Design review of the part built by this model. Coordinates are the model's own, in mm. Face numbers are marked on the shaded views. A direction names the side the tool comes from. Round coordinates to 2 decimals unless told otherwise and drop trailing zeros. Loops run counter-clockwise (first coordinate to the right, second up) from the corner with the lowest first, then second, coordinate; pieces in that order, holes last. Notation, with made-up numbers: (-28.5, 82.25) - (-6.5, 82.25) arc R10 cw to (-6.5, 100.25) - close; hole circle Ø6 at (-25.75, 36.5). An arc over 180 degrees is marked (long way). Return JSON: item names as keys, results as strings. Group by question number.
(1) The part is to be moulded in two halves that separate along X. For the marked faces 3, 4 and 5, say which applies: pulls with the +X half, pulls with the -X half, needs draft (parallel to the pull), parting line crosses it, or undercut.
(2) We need section D-D, the plane z = -13.5. Write out the cut boundary in (x, y), and give its area (3 significant figures).
(3) We need section B-B, the plane y = 20.25. Write out the cut boundary in (x, z).
(4) Wall thickness on L1, parallel to X at y = 25.7, z = 13.5; L2, parallel to X at y = 5, z = -13.5; L3, parallel to X at y = 9, z = 0: over which ranges is each line inside the solid? List them lowest first. Write a range as [from, to].
(5) For the marked faces 1 and 2, list the 3-axis set-ups (+Z, -Z, +X, -X, +Y, -Y) from which the entire face can be reached by the end or side of a thin tool; tool diameter is ignored.
(6) We need section A-A, the plane z = 0. Write out the cut boundary in (x, y).
(7) We need section C-C, the plane x = 0. Give the number of separate pieces and of enclosed holes in the cut face, and give its area (3 significant figures).
(8) Clearance check with flat-ended pins moving along their axes: pin 1 (1.5 mm diameter, centred on y = 20, z = -22.5, fed in from +X); pin 2 (11 mm diameter, centred on x = -2, z = -29, fed in from +Y); pin 3 (10 mm diameter, centred on x = 8.5, z = -0.5, fed in from +Y); pin 4 (10 mm diameter, centred on y = 26, z = -17, fed in from -X). State where each tip first meets the part, or that it passes through.
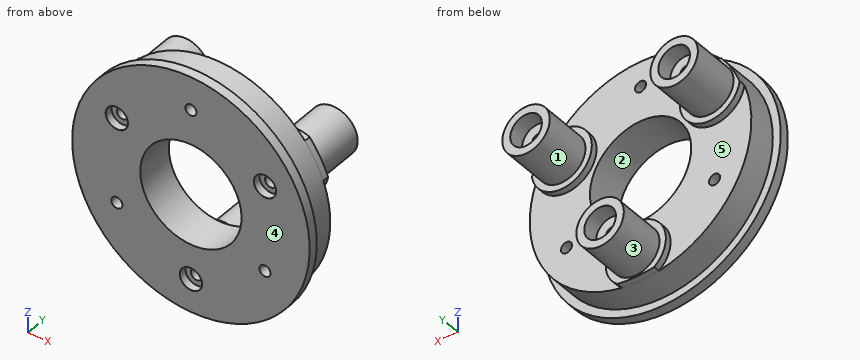
from build123d import *

# Parameters (mm, degrees)
SKETCH1_R                                     = 37.5
BOSS_EXTRUDE1_DEPTH                           = 3
SKETCH1_3_R                                   = 35
BOSS_EXTRUDE2_DEPTH                           = 12
SKETCH13_R                                    = 16
CUT_EXTRUDE6_DEPTH                            = 55.373706881
BOSS_EXTRUDE9_DEPTH                           = 2
SKETCH25_R                                    = 7.5
BOSS_EXTRUDE10_DEPTH                          = 15
SKETCH26_R                                    = 5
CUT_EXTRUDE9_DEPTH                            = 5
CBORE_FOR_M3_PAN_HEAD_MACHINE_SCREW1_AT_COUNT = 2
CBORE_FOR_M3_PAN_HEAD_MACHINE_SCREW1_AT_PITCH = 46.765371804
CBORE_FOR_M3_PAN_HEAD_MACHINE_SCREW1_2_COUNT  = 2
CBORE_FOR_M3_PAN_HEAD_MACHINE_SCREW1_2_PITCH  = 46.765371804
SKETCH29_R                                    = 1.75
CUT_EXTRUDE10_DEPTH                           = 56.691112397


with BuildPart() as part:
    # Sketch1 → Boss-Extrude1 (new body)
    with BuildSketch(Plane(origin=(0, 0, 0), x_dir=(1, 0, 0), z_dir=(0, 1, 0))):
        with Locations(Location((0, 0, 0), (0, 0, 270))):
            Circle(SKETCH1_R)
    extrude(amount=BOSS_EXTRUDE1_DEPTH)

    # Sketch1_3 → Boss-Extrude2 (add)
    with BuildSketch(Plane(origin=(0, 0, 0), x_dir=(1, 0, 0), z_dir=(0, 1, 0))):
        with Locations(Location((0, 0, 0), (0, 0, 270))):
            Circle(SKETCH1_3_R)
    extrude(amount=BOSS_EXTRUDE2_DEPTH)

    # Sketch13 → Cut-Extrude6 (cut, through all)
    with BuildSketch(Plane(origin=(0, 12, 0), x_dir=(1, 0, 0), z_dir=(0, 1, 0))):
        with Locations(Location((0, 0, 0), (0, 0, 270))):
            Circle(SKETCH13_R)
    extrude(amount=-CUT_EXTRUDE6_DEPTH, mode=Mode.SUBTRACT)

    # Sketch24 → Boss-Extrude9 (add)
    with BuildSketch(Plane(origin=(0, 12, 0), x_dir=(1, 0, 0), z_dir=(0, 1, 0))):
        with BuildLine():
            ThreePointArc((5.813043417, 34.513888889), (0, 35), (-5.813043417, 34.513888889))
            ThreePointArc((-5.813043417, 34.513888889), (0, 17.5), (5.813043417, 34.513888889))
        make_face()
        with BuildLine():
            ThreePointArc((-26.983382853, -22.291187717), (-15.155444566, -8.75), (-32.79642627, -12.222701172))
            ThreePointArc((-32.79642627, -12.222701172), (-30.310889132, -17.5), (-26.983382853, -22.291187717))
        make_face()
        with BuildLine():
            ThreePointArc((26.983382853, -22.291187717), (30.310889132, -17.5), (32.79642627, -12.222701172))
            ThreePointArc((32.79642627, -12.222701172), (15.155444566, -8.75), (26.983382853, -22.291187717))
        make_face()
    extrude(amount=BOSS_EXTRUDE9_DEPTH)

    # Sketch25 → Boss-Extrude10 (add)
    with BuildSketch(Plane(origin=(0, 14, 0), x_dir=(1, 0, 0), z_dir=(0, 1, 0))):
        with Locations(Location((0, 27, 0), (0, 0, 270))):
            Circle(SKETCH25_R)
        with Locations(Location((23.382685902, -13.5, 0), (0, 0, 270))):
            Circle(SKETCH25_R)
        with Locations(Location((-23.382685902, -13.5, 0), (0, 0, 270))):
            Circle(SKETCH25_R)
    extrude(amount=BOSS_EXTRUDE10_DEPTH)

    # Sketch26 → Cut-Extrude9 (cut)
    with BuildSketch(Plane(origin=(0, 29, 0), x_dir=(1, 0, 0), z_dir=(0, 1, 0))):
        with Locations(Location((0, 27, 0), (0, 0, 270))):
            Circle(SKETCH26_R)
        with Locations(Location((23.382685902, -13.5, 0), (0, 0, 270))):
            Circle(SKETCH26_R)
        with Locations(Location((-23.382685902, -13.5, 0), (0, 0, 270))):
            Circle(SKETCH26_R)
    extrude(amount=-CUT_EXTRUDE9_DEPTH, mode=Mode.SUBTRACT)

    # Sketch28 → CBORE for M3 Pan Head Machine Screw1 (revolve, cut)
    with BuildSketch(Plane(origin=(0, 0, -27), x_dir=(0, 0, -1), z_dir=(1, 0, 0))):
        Polygon((0, 0), (0, 29), (1.8, 29), (1.8, 2.4), (3.5, 2.4), (3.5, 0.025), (3.525, 0), align=None)
    cbore_for_m3_pan_head_machine_screw1 = revolve(axis=Axis((0, -6.35, -27), (0, 1, 0)), mode=Mode.SUBTRACT)

    # CBORE for M3 Pan Head Machine Screw1 at: CBORE for M3 Pan Head Machine Screw1 ×2
    with Locations(*[Vector(-0.5000000000000369, 0, 0.8660254037844174) * (i * CBORE_FOR_M3_PAN_HEAD_MACHINE_SCREW1_AT_PITCH) for i in range(1, CBORE_FOR_M3_PAN_HEAD_MACHINE_SCREW1_AT_COUNT)]):
        add(cbore_for_m3_pan_head_machine_screw1, mode=Mode.SUBTRACT)

    # CBORE for M3 Pan Head Machine Screw1 2: CBORE for M3 Pan Head Machine Screw1 ×2
    with Locations(*[Vector(0.49999999999996353, 0, 0.8660254037844598) * (i * CBORE_FOR_M3_PAN_HEAD_MACHINE_SCREW1_2_PITCH) for i in range(1, CBORE_FOR_M3_PAN_HEAD_MACHINE_SCREW1_2_COUNT)]):
        add(cbore_for_m3_pan_head_machine_screw1, mode=Mode.SUBTRACT)

    # Sketch29 → Cut-Extrude10 (cut, through all)
    with BuildSketch(Plane(origin=(0, 12, 0), x_dir=(1, 0, 0), z_dir=(0, 1, 0))):
        with Locations(Location((23.382685902, 13.5, 0), (0, 0, 270))):
            Circle(SKETCH29_R)
        with Locations(Location((0, -27, 0), (0, 0, 270))):
            Circle(SKETCH29_R)
        with Locations(Location((-23.382685902, 13.5, 0), (0, 0, 270))):
            Circle(SKETCH29_R)
    extrude(amount=-CUT_EXTRUDE10_DEPTH, mode=Mode.SUBTRACT)


solid = part.part
Solutions:
{
 "1": {"face 3": "parting line crosses it", "face 4": "needs draft", "face 5": "undercut"},
 "2": {"outline": "(-34.99, 0) - (-25.13, 0) - (-25.13, 12) - (-32.29, 12) - (-32.29, 3) - (-34.99, 3) - close; (-21.63, 0) - (-8.59, 0) - (-8.59, 12) - (-21.63, 12) - close; (8.59, 0) - (21.63, 0) - (21.63, 12) - (8.59, 12) - close; (25.13, 0) - (34.99, 0) - (34.99, 3) - (32.29, 3) - (32.29, 12) - (25.13, 12) - close", "area": "501 mm^2"},
 "3": {"outline": "circle Ø15 at (-23.38, 13.5); circle Ø15 at (0, -27); circle Ø15 at (23.38, 13.5); hole circle Ø3.6 at (-23.38, 13.5); hole circle Ø3.6 at (0, -27); hole circle Ø3.6 at (23.38, 13.5)"},
 "4": {"L1": "[-30.88, -28.38], [-18.38, -15.88], [15.88, 18.38], [28.38, 30.88]", "L2": "[-32.29, -25.13], [-21.63, -8.59], [8.59, 21.63], [25.13, 32.29]", "L3": "[-35, -16], [16, 35]"},
 "5": {"face 1": "+Y", "face 2": "+Y, -Y"},
 "6": {"outline": "(-37.5, 0) - (-16, 0) - (-16, 12) - (-35, 12) - (-35, 3) - (-37.5, 3) - close; (16, 0) - (37.5, 0) - (37.5, 3) - (35, 3) - (35, 12) - (16, 12) - close"},
 "7": {"separate pieces": "4", "enclosed holes": "0", "area": "544 mm^2"},
 "8": {"pin 1": "x = 6.5", "pin 2": "y = 29", "pin 3": "through", "pin 4": "x = -5.59"}
}
